For this review, take the finished solid that the model builds, in its own axes (mm). Face numbers are marked on the shaded views. A direction names the side the tool comes from. Give positions to 0.01 mm unless a question says otherwise; leave off trailing zeros. Loops run counter-clockwise (first coordinate to the right, second up) from the corner with the lowest first, then second, coordinate; pieces in that order, holes last. Notation, with made-up numbers: (1, -20.75) - (32, -20.75) arc R20 cw to (32, -11.75) - close; hole circle Ø7 at (52, 70.25). An arc over 180 degrees is marked (long way). Answer as CSV lines item,"result".
from build123d import *

# Parameters (mm, degrees)
SKETCH1_W           = 79.713100929
SKETCH1_H           = 188.030607332
SKETCH1_W_2         = 54.313100929
SKETCH1_H_2         = 162.630607332
EXTRUDE_THIN1_DEPTH = 1.5875
EXTRUDE_THIN2_START = -179.324
SKETCH1_3_W         = 79.713100929
SKETCH1_3_H         = 188.030607332
SKETCH1_3_W_2       = 54.313100929
SKETCH1_3_H_2       = 162.630607332
EXTRUDE_THIN2_DEPTH = 1.5875
SKETCH2_W           = 79.713100929
SKETCH2_H           = 12.7
BOSS_EXTRUDE3_DEPTH = 25.4
BOSS_EXTRUDE4_START = -182.499
SKETCH2_2_W         = 79.713100929
SKETCH2_2_H         = 12.7
BOSS_EXTRUDE4_DEPTH = 25.4
SKETCH3_W           = 117.076053855
SKETCH3_H           = 196.691722882
CUT_EXTRUDE1_DEPTH  = 291.300056469


with BuildPart() as part:
    # Sketch1 → Extrude-Thin1 (new body)
    with BuildSketch(Plane(origin=(179.324, 0, 0), x_dir=(0, 0, -1), z_dir=(1, 0, 0))):
        with Locations((39.856550465, 94.015303666)):
            Rectangle(SKETCH1_W, SKETCH1_H)
        with Locations((39.856550465, 94.015303666)):
            Rectangle(SKETCH1_W_2, SKETCH1_H_2, mode=Mode.SUBTRACT)
    extrude(amount=EXTRUDE_THIN1_DEPTH)

    # Sketch2 → Boss-Extrude3 (add)
    with BuildSketch(Plane(origin=(180.9115, 0, 0), x_dir=(0, 0, -1), z_dir=(1, 0, 0))):
        with Locations((39.856550465, 6.35)):
            Rectangle(SKETCH2_W, SKETCH2_H)
    extrude(amount=BOSS_EXTRUDE3_DEPTH)


with BuildPart() as body_2:
    # Sketch1<3> → Extrude-Thin2 (new body)
    with BuildSketch(Plane(origin=(179.324, 0, 0), x_dir=(0, 0, -1), z_dir=(1, 0, 0)).offset(EXTRUDE_THIN2_START)):
        with Locations((39.856550465, 94.015303666)):
            Rectangle(SKETCH1_3_W, SKETCH1_3_H)
        with Locations((39.856550465, 94.015303666)):
            Rectangle(SKETCH1_3_W_2, SKETCH1_3_H_2, mode=Mode.SUBTRACT)
    extrude(amount=-EXTRUDE_THIN2_DEPTH)

    # Sketch2<2> → Boss-Extrude4 (add)
    with BuildSketch(Plane(origin=(180.9115, 0, 0), x_dir=(0, 0, -1), z_dir=(1, 0, 0)).offset(BOSS_EXTRUDE4_START)):
        with Locations((39.856550465, 6.35)):
            Rectangle(SKETCH2_2_W, SKETCH2_2_H)
    extrude(amount=-BOSS_EXTRUDE4_DEPTH)

    # Sketch3 → Cut-Extrude1 (cut, through all)
    with BuildSketch(Plane(origin=(0, 0, 0), x_dir=(0, 0, -1), z_dir=(1, 0, 0))):
        with Locations((58.538026928, 98.345861441)):
            Rectangle(SKETCH3_W, SKETCH3_H)
    extrude(amount=-CUT_EXTRUDE1_DEPTH, mode=Mode.SUBTRACT)


solid = part.part
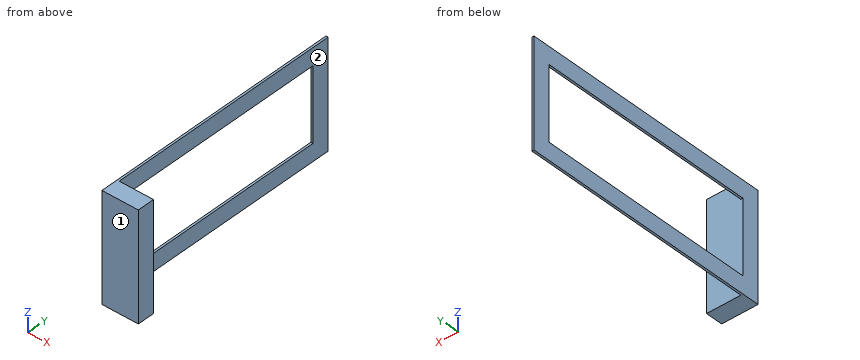
1) Wall thickness on line 1 (Y direction, x = 192.75, z = -28); line 2 (X direction, y = 23, z = -70): over which ranges is each line inside the solid? List them lowest first. Write a range as from..to.
From the geometry:
line 1,"y = 0..12.7"
line 2,"x = 179.32..180.91"
2) Consider section A-A on y = 42. Write out the cut boundary in (x, z).
From the geometry:
outline,"(179.32, -79.71) - (180.91, -79.71) - (180.91, -67.01) - (179.32, -67.01) - close; (179.32, -12.7) - (180.91, -12.7) - (180.91, 0) - (179.32, 0) - close"
3) Machinability: for the marked faces 1 and 2, which of the approach directions +Z, -Z, +X, -X, +Y, -Y give a long, thin tool a straight path to every point of the face, cutting with its end or side? Answer none if there is none.
From the geometry:
face 1,"+Z, -Z, +X, -X, -Y"
face 2,"+Z, -Z, +X, +Y"
4) Consider section D-D on x = 199.75. Write out the cut boundary in (y, z), and give its area (3 significant figures).
From the geometry:
outline,"(0, -79.71) - (12.7, -79.71) - (12.7, 0) - (0, 0) - close"
area,"1,010 mm^2"
5) Consider section B-B on z = -22.5. Write out the cut boundary in (x, y), and give its area (3 significant figures).
From the geometry:
outline,"(179.32, 0) - (206.31, 0) - (206.31, 12.7) - (179.32, 12.7) - close; (179.32, 175.33) - (180.91, 175.33) - (180.91, 188.03) - (179.32, 188.03) - close"
area,"363 mm^2"
6) Consider section C-C on z = -9.5. Write out the cut boundary in (x, y).
From the geometry:
outline,"(179.32, 0) - (206.31, 0) - (206.31, 12.7) - (180.91, 12.7) - (180.91, 188.03) - (179.32, 188.03) - close"
7) Insertion check: P1, Ø3, axis at x = 192.5, z = -70, coming from the +Y side. The pin has a flat end and moves straight along its axis. Give the tip position at first contact, or say it passes through.
From the geometry:
P1,"stops at y = 12.7"
